Could you check a few things on this model? Use its own coordinates, in mm. A direction names the side the tool comes from. Round coordinates to 2 decimals unless told otherwise and drop trailing zeros. Loops run counter-clockwise (first coordinate to the right, second up) from the corner with the lowest first, then second, coordinate; pieces in that order, holes last. Notation, with made-up numbers: M 47,86.25 L 70,86.25 A15 ccw 70,102.25 Z; hole C 16,14 d9. An arc over 180 degrees is marked long. One line per item, written item: value. Start each with the question number.
Q1. Imagine slicing it at B-B (z = 1.7). Please give me the cut outline in (x, y) (3 decimals), then the cut area to 3 significant figures.
Q2. Please list where these lines run through material, in increasing order: line 1 along Y through (x, z) = (0, 3.55) (3 decimals); line 2 along Y through (x, z) = (1, 3.05) (3 decimals); line 3 along X through (y, z) = (9, 2.8) (3 decimals).
Q3. Imagine slicing it at A-A (x = 7). Please give me the cut outline in (y, z) (1 decimal), then the cut area to 3 significant figures.
Q4. Imagine slicing it at D-D (x = 10.5). Please give me the cut outline in (y, z) (1 decimal), then the cut area to 3 significant figures.
Q5. Thinking about a two-plate mould opening in Y: for faces 1 (the face through (1.354, -10.735, 2.348)), 2 (the face through (15, 14, 0)), 3 (the face through (-9.4, 9.525, 3.7)), 4 (the face through (-9.6, -9.525, 3.7)), which applies, released by +Y, released by -Y, zero draft, split by the parting line, or undercut?
Q6. Which directions (+Z, -Z, +X, -X, +Y, -Y) give clear straight access to the entire face, cutting with the end or side of a thin tool? Please do faces 5 (the face through (11, 12.7, 3)), 6 (the face through (-3.175, 13, 2)), 7 (the face through (15.875, -14, 2)).
Q7. I'm going to push a flat-ended pin straight in: pin 1 Ø2 at (y, z) = (7, 3.5) entering from +X. Where does the tip first touch, or does it pass through?
from build123d import *

# Parameters (mm, degrees)
F0_R     = 2.54
F1_DEPTH = 4.7625
F2_R     = 0.79375
F4_DEPTH = 25.401
F6_DEPTH = 31.751
F8_DEPTH = 0.0254


with BuildPart() as f1:
    # F0 (on Top) → F1 (new body)
    with BuildSketch(Plane.XY):
        Polygon((15.875, 12.7), (15.875, 15.875), (-3.175, 15.875), (-3.175, 9.525), (-15.875, 9.525), (-15.875, -9.525), (-3.175, -9.525), (-3.175, -15.875), (15.875, -15.875), (15.875, -12.7), (6.35, -12.7), (6.35, 12.7), align=None)
        with Locations((1.905, -8.255)):
            Circle(F0_R, mode=Mode.SUBTRACT)
        with Locations((1.905, 8.255)):
            Circle(F0_R, mode=Mode.SUBTRACT)
    extrude(amount=F1_DEPTH)

    # F2
    f2_edges = [f1.edges().sort_by_distance(p)[0] for p in [
        (-9.525, 9.525, 4.7625),
        (-9.525, -9.525, 4.7625),
        (6.35, 15.875, 4.7625),
        (11.1125, 12.7, 4.7625),
        (6.35, 0, 4.7625),
        (15.875, 14.2875, 4.7625),
        (11.1125, -12.7, 4.7625),
        (15.875, -14.2875, 4.7625),
        (6.35, -15.875, 4.7625),
        (-3.175, -12.7, 4.7625),
        (-15.875, 0, 4.7625),
        (-3.175, 12.7, 4.7625),
    ]]
    fillet(f2_edges, radius=F2_R)

    # F3 (on face) → F4 (cut, through all)
    with BuildSketch(Plane.XZ.offset(9.525)):
        with BuildLine():
            Line((-12.7, 0), (-6.35, 0))
            ThreePointArc((-6.35, 0), (-9.525, 3.175), (-12.7, 0))
        make_face()
    extrude(amount=-F4_DEPTH, mode=Mode.SUBTRACT)

    # F5 (on face) → F6 (cut, through all)
    with BuildSketch(Plane.XZ.offset(15.875)):
        with BuildLine():
            Line((8.41375, 0), (13.17625, 0))
            ThreePointArc((13.17625, 0), (10.795, 2.38125), (8.41375, 0))
        make_face()
    extrude(amount=-F6_DEPTH, mode=Mode.SUBTRACT)

    # F7 (on face) → F8 (cut)
    with BuildSketch(Plane.XY.offset(4.7625)):
        Polygon((-10.099244, -6.511544), (-10.099244, -7.751831), (-9.488716, -7.751831), (-9.488716, -6.511544), (-7.894327, -6.511544), (-7.894327, -6.002771), (-9.488716, -6.002771), (-9.488716, -4.706035), (-7.894327, -4.706035), (-7.894327, -4.197262), (-9.488716, -4.197262), (-9.488716, -3.179715), (-7.894327, -3.179715), (-7.894327, -2.670942), (-9.488716, -2.670942), (-9.488716, -1.780588), (-7.894327, -1.780588), (-7.894327, -1.322692), (-9.488716, -1.322692), (-9.488716, -0.228829), (-7.894327, -0.228829), (-7.894327, 0.228829), (-9.488716, 0.228829), (-9.488716, 1.545488), (-7.894327, 1.545488), (-7.894327, 2.003385), (-9.488716, 2.003385), (-9.488716, 3.542424), (-7.856169, 3.542424), (-7.856169, 4.000321), (-9.488716, 4.000321), (-9.488716, 5.580434), (-7.892068, 5.580434), (-7.892068, 6.035207), (-9.488716, 6.035207), (-9.488716, 7.751831), (-10.099244, 7.751831), (-10.099244, 6.035207), (-11.719226, 6.035207), (-11.719226, 5.580434), (-10.099244, 5.580434), (-10.099244, 4.000321), (-11.646531, 4.000321), (-11.646531, 3.542424), (-10.099244, 3.542424), (-10.099244, 2.003385), (-11.659251, 2.003385), (-11.659251, 1.545488), (-10.099244, 1.545488), (-10.099244, 0.228829), (-11.693633, 0.228829), (-11.693633, -0.228829), (-10.099244, -0.228829), (-10.099244, -1.322692), (-11.693633, -1.322692), (-11.693633, -1.780588), (-10.099244, -1.780588), (-10.099244, -2.670942), (-11.693633, -2.670942), (-11.693633, -3.179715), (-10.099244, -3.179715), (-10.099244, -4.197262), (-11.693633, -4.197262), (-11.693633, -4.706035), (-10.099244, -4.706035), (-10.099244, -6.002771), (-11.693633, -6.002771), (-11.693633, -6.511544), align=None)
    extrude(amount=-F8_DEPTH, mode=Mode.SUBTRACT)


solid = f1.part
Report:
1. outline: M -15.875,-9.525 L -12.207,-9.525 L -12.207,9.525 L -15.875,9.525 Z; M -6.843,-9.525 L -3.175,-9.525 L -3.175,-15.875 L 9.128,-15.875 L 9.128,-12.7 L 6.35,-12.7 L 6.35,12.7 L 9.128,12.7 L 9.128,15.875 L -3.175,15.875 L -3.175,9.525 L -6.843,9.525 Z; M 12.462,-15.875 L 15.875,-15.875 L 15.875,-12.7 L 12.462,-12.7 Z; M 12.462,12.7 L 15.875,12.7 L 15.875,15.875 L 12.462,15.875 Z; hole C 1.905,-8.255 d5.08; hole C 1.905,8.255 d5.08
1. area: 441 mm²
2. line 1: y = -15.875 to -9.935, -6.575 to 6.575, 9.935 to 15.875
2. line 2: y = -15.875 to -10.628, -5.882 to 5.882, 10.628 to 15.875
2. line 3: x = -15.875 to -11.022, -8.028 to -0.523, 4.333 to 6.35
3. outline: M -15.9,0 L -12.7,0 L -12.7,4 A0.8 ccw -13.5,4.8 L -15.1,4.8 A0.8 ccw -15.9,4 Z; M 12.7,0 L 15.9,0 L 15.9,4 A0.8 ccw 15.1,4.8 L 13.5,4.8 A0.8 ccw 12.7,4 Z
3. area: 29.7 mm²
4. outline: M -15.9,2.4 L -12.7,2.4 L -12.7,4 A0.8 ccw -13.5,4.8 L -15.1,4.8 A0.8 ccw -15.9,4 Z; M 12.7,2.4 L 15.9,2.4 L 15.9,4 A0.8 ccw 15.1,4.8 L 13.5,4.8 A0.8 ccw 12.7,4 Z
4. area: 14.7 mm²
5. face 1: undercut
5. face 2: zero draft
5. face 3: released by +Y
5. face 4: released by -Y
6. face 5: +Z, -Z, +X
6. face 6: +Z, -Z, -X, +Y
6. face 7: +Z, -Z, +X, +Y, -Y
7. pin 1: stops at x = 6.35
